Input: part model. Units: mm. Frame: model coordinates. A direction names the side the tool comes from. Round coordinates to 2 decimals unless told otherwise and drop trailing zeros. Order: outer loops, then holes, each group sorted by start corner. A loop starts at its lowest first (then second) coordinate and runs counter-clockwise, first axis right, second up. Notation, with made-up numbers: M -11.5,-4.75 L 35.5,-4.75 A20 cw 35.5,16.25 Z; hole C -31,70 d8. An arc over 180 degrees is marked long. One line per question, with ' | ' between items.
```python
from build123d import *

# Parameters (mm, degrees)
ESBO_O1_R                = 5
RESSALTO_EXTRUS_O1_DEPTH = 54.2
ESBO_O2_R                = 5
ESBO_O2_R_2              = 3.3
CORTE_EXTRUS_O1_DEPTH    = 8


with BuildPart() as part:
    # Esboço1 → Ressalto-extrusão1 (new, symmetric)
    with BuildSketch(Plane(origin=(0, 0, 0), x_dir=(1, 0, 0), z_dir=(0, 1, 0))):
        with Locations(Location((0, 0, 0), (0, 0, 90))):
            Circle(ESBO_O1_R)
    extrude(amount=RESSALTO_EXTRUS_O1_DEPTH, both=True)

    # Esboço2 → Corte-extrusão1 (cut)
    with BuildSketch(Plane(origin=(0, 54.2, 0), x_dir=(1, 0, 0), z_dir=(0, 1, 0))):
        with Locations(Location((0, 0, 0), (0, 0, 90))):
            Circle(ESBO_O2_R)
        with Locations(Location((0, 0, 0), (0, 0, 270))):
            Circle(ESBO_O2_R_2, mode=Mode.SUBTRACT)
    corte_extrus_o1 = extrude(amount=-CORTE_EXTRUS_O1_DEPTH, mode=Mode.SUBTRACT)

    # Espelhar1: Corte-extrusão1 across plane
    add(corte_extrus_o1.mirror(Plane.ZX), mode=Mode.SUBTRACT)


solid = part.part
```
Item 1: Section query B-B, the plane x = 0. Return loops of the section in (y, z).
Report:
outline: M -54.2,-3.3 L -46.2,-3.3 L -46.2,-5 L 46.2,-5 L 46.2,-3.3 L 54.2,-3.3 L 54.2,3.3 L 46.2,3.3 L 46.2,5 L -46.2,5 L -46.2,3.3 L -54.2,3.3 Z
Item 2: Access query for faces 1 (the flat face through (3.3, -46.2, 1.2)), 2 (the cylindrical face through (-2.008, 50.256, -2.619)), 3 (the flat face through (0, 54.2, 0)). Directions: +Z, -Z, +X, -X, +Y, -Y. A direction counts if a zero-diameter tool reaches every point of the face in a straight line with its end or side. Return the directions, or none.
Report:
face 1: -Y | face 2: +Y | face 3: +Z, -Z, +X, -X, +Y
Item 3: Line query: line 1 along Z through (x, y) = (-0.25, -47); line 2 along Z through (x, y) = (0.25, -18); line 3 along Y through (x, z) = (3.75, 0). Output: solid intervals per line, ascending. Write a range as from..to.
Report:
line 1: -3.29..3.29 | line 2: -4.99..4.99 | line 3: -46.2..46.2
Item 4: Section query A-A, the plane z = 0. Return loops of the section in (x, y), plus the area to 3 significant figures.
Report:
outline: M -5,-46.2 L -3.3,-46.2 L -3.3,-54.2 L 3.3,-54.2 L 3.3,-46.2 L 5,-46.2 L 5,46.2 L 3.3,46.2 L 3.3,54.2 L -3.3,54.2 L -3.3,46.2 L -5,46.2 Z | area: 1,030 mm²
Item 5: Section query C-C, the plane y = 37. Return loops of the section in (x, z), plus the area to 3 significant figures.
Report:
outline: C 0,0 d10 | area: 78.5 mm²
Item 6: First-contact query: pin 1 (1.5 mm diameter, centred on y = 21.5, z = 1, fed in from +X); pin 2 (2 mm diameter, centred on x = 1.5, y = 27, fed in from +Z); pin 3 (2 mm diameter, centred on x = 1.5, y = -26.5, fed in from -Z). Flat tips, straight axial feed; report the tip coordinate or a pass-through.
Report:
pin 1: x = 4.99 | pin 2: z = 4.97 | pin 3: z = -4.97
